```python
from build123d import *

# Parameters (mm, degrees)
F0_W             = 25
F0_H             = 25
F0_R             = 4
F1_DEPTH         = 3
F2_W             = 10
F2_H             = 0.5
F3_DEPTH         = 6.001
F3_COPIES2_COUNT = 2
F4_R             = 0.24999


# Not quite as in the source:
# - a fillet or chamfer is up to 0.001 mm smaller than in the source, because OpenCascade refuses the exact size
# - a pattern or mirror of a feature is missing from the dataset's text; its kind, count and spacing are read off the source's solid


with BuildPart() as f1:
    # F0 (on Front) → F1 (new body, symmetric)
    with BuildSketch(Plane.XZ):
        Rectangle(F0_W, F0_H)
        Circle(F0_R, mode=Mode.SUBTRACT)
    extrude(amount=F1_DEPTH, both=True)

    # F2 (on face) → F3 (cut, through all)
    with BuildSketch(Plane.XZ.offset(3)):
        with BuildLine():
            ThreePointArc((-4.2426406871, 4.2426406871), (-2.2961005942, 5.5432771951), (0, 6))
            Line((0, 6), (0, 6.5))
            ThreePointArc((0, 6.5), (-1.96297305, 6.1965100504), (-3.7426406871, 5.3143805554))
            Line((-3.7426406871, 5.3143805554), (-3.7426406871, 9.75))
            Line((-3.7426406871, 9.75), (-4.2426406871, 9.75))
            Line((-4.2426406871, 9.75), (-4.2426406871, 4.2426406871))
        make_face()
        with BuildLine():
            Line((-6.5, 0), (-6, 0))
            ThreePointArc((-6, 0), (-5.6105188763, 2.1265177965), (-4.4926406871, 3.9769560793))
            Line((-4.4926406871, 3.9769560793), (-4.4926406871, 9.75))
            Line((-4.4926406871, 9.75), (-10, 9.75))
            Line((-10, 9.75), (-10, 9.25))
            Line((-10, 9.25), (-4.9926406871, 9.25))
            Line((-4.9926406871, 9.25), (-4.9926406871, 4.1621555677))
            ThreePointArc((-4.9926406871, 4.1621555677), (-6.1115531768, 2.2133498971), (-6.5, 0))
        make_face()
        with Locations((-5, 10.25)):
            Rectangle(F2_W, F2_H)
    f3 = extrude(amount=-F3_DEPTH, mode=Mode.SUBTRACT)

    # F3_copies: F3 across plane
    add(f3.mirror(Plane(origin=(0, 0, 0), x_dir=(-1, 0, 0), z_dir=(0, 0, -1))), mode=Mode.SUBTRACT)

    # F3_copies1: F3 across plane
    add(f3.mirror(Plane(origin=(0, 0, 0), x_dir=(0, 0, 1), z_dir=(1, 0, 0))), mode=Mode.SUBTRACT)

    # F3_copies2: F3 ×2 about axis
    f3_copies2_axis = Axis((0, 0, 0), (0, 1, 0))
    for i in range(1, F3_COPIES2_COUNT):
        add(f3.rotate(f3_copies2_axis, i * 360 / F3_COPIES2_COUNT), mode=Mode.SUBTRACT)

    # F4 (radius 0.25 in the source; OpenCascade refuses exactly that, so slightly less here)
    f4_edges = [f1.edges().sort_by_distance(p)[0] for p in [
        (-10, 0, 10),
        (-4.492641, 0, 9.75),
        (-4.492641, 0, 3.976956),
        (-4.242641, 0, 4.242641),
        (-10, 0, 10.5),
        (-4.242641, 0, 9.75),
        (-10, 0, 9.25),
        (-10, 0, 9.75),
        (-3.742641, 0, 9.75),
        (-3.742641, 0, 5.314381),
        (10, 0, 10),
        (10, 0, 10.5),
        (10, 0, 9.25),
        (10, 0, 9.75),
        (4.492641, 0, 9.75),
        (4.492641, 0, 3.976956),
        (4.492641, 0, -3.976956),
        (4.492641, 0, -9.75),
        (10, 0, -9.75),
        (10, 0, -9.25),
        (4.242641, 0, 4.242641),
        (4.242641, 0, 9.75),
        (3.742641, 0, 9.75),
        (3.742641, 0, 5.314381),
        (-10, 0, -9.25),
        (-10, 0, -9.75),
        (-4.492641, 0, -9.75),
        (-4.492641, 0, -3.976956),
        (-3.742641, 0, -9.75),
        (-3.742641, 0, -5.314381),
        (3.742641, 0, -5.314381),
        (3.742641, 0, -9.75),
        (4.242641, 0, -9.75),
        (4.242641, 0, -4.242641),
        (-4.242641, 0, -4.242641),
        (-4.242641, 0, -9.75),
        (10, 0, -10),
        (10, 0, -10.5),
        (-10, 0, -10),
        (-10, 0, -10.5),
    ]]
    fillet(f4_edges, radius=F4_R)


solid = f1.part
```
Work out the finished part from the listing and answer in its coordinate system (mm). A direction names the side the tool comes from. Give positions to 0.01 mm unless a question says otherwise; leave off trailing zeros. Write each loop counter-clockwise with the first axis right and the second up, starting at its lowest first coordinate (ties: lowest second). Pieces come first, ordered by that corner, then holes. Notation, with made-up numbers: (-11, 84.25) -> (17, 84.25) arc R12 ccw to (17, 106.25) -> close; hole circle Ø8 at (25.25, 8.25). An arc over 180 degrees is marked (long way). Write each question's results on one line, items separated by ' | '.
1. Find section A-A on z = 7.5. Determine the outline of the cut face in (x, y).
Data:
outline: (-12.5, -3) -> (-4.99, -3) -> (-4.99, 3) -> (-12.5, 3) -> close; (-4.49, -3) -> (-4.24, -3) -> (-4.24, 3) -> (-4.49, 3) -> close; (-3.74, -3) -> (3.74, -3) -> (3.74, 3) -> (-3.74, 3) -> close; (4.24, -3) -> (4.49, -3) -> (4.49, 3) -> (4.24, 3) -> close; (4.99, -3) -> (12.5, -3) -> (12.5, 3) -> (4.99, 3) -> close
2. Find section D-D on y = 0.35. Give the number of separate pieces and of enclosed holes in the cut face, and give its area (3 significant figures).
Data:
separate pieces: 1 | enclosed holes: 7 | area: 506 mm^2
3. Find section B-B on x = -1.75. Determine the outline of the cut face in (y, z).
Data:
outline: (-3, -12.5) -> (3, -12.5) -> (3, -10.5) -> (-3, -10.5) -> close; (-3, -10) -> (3, -10) -> (3, -6.26) -> (-3, -6.26) -> close; (-3, -5.74) -> (3, -5.74) -> (3, -3.6) -> (-3, -3.6) -> close; (-3, 3.6) -> (3, 3.6) -> (3, 5.74) -> (-3, 5.74) -> close; (-3, 6.26) -> (3, 6.26) -> (3, 10) -> (-3, 10) -> close; (-3, 10.5) -> (3, 10.5) -> (3, 12.5) -> (-3, 12.5) -> close
4. A tool of negligible diameter and unlimited length cuts with its end or side. For faces 1 (the flat face through (-3, 3, 3)), 2 (the flat face through (7, 0, 9.25)), from which of +Z, -Z, +X, -X, +Y, -Y can it reach the whole face along a straight path? Write none if from no direction.
Data:
face 1: +Z, -Z, +X, -X, +Y | face 2: +Y, -Y
5. Find section C-C on z = -1.5. Determine the outline of the cut face in (x, y).
Data:
outline: (-12.5, -3) -> (-6.32, -3) -> (-6.32, 3) -> (-12.5, 3) -> close; (-5.81, -3) -> (-3.71, -3) -> (-3.71, 3) -> (-5.81, 3) -> close; (3.71, -3) -> (5.81, -3) -> (5.81, 3) -> (3.71, 3) -> close; (6.32, -3) -> (12.5, -3) -> (12.5, 3) -> (6.32, 3) -> close
6. Determine the mould class of faces 3 (the flat face through (0, 0, 10)), 4 (the flat face through (12.5, 0, 0)) for opening direction Z: +Z half, -Z half, draft (parallel to the pull), parting line (faces both ways), or undercut.
Data:
face 3: undercut | face 4: draft
7. Straight lines are drawn through the part: L1, parallel to X at y = 2.55, z = 7.5; L2, parallel to Z at x = 9.5, y = -1.2; L3, parallel to X at y = -0.65, z = -0.25. For each, find the intervals that lie inside material, in ascending order.
Data:
L1: -12.5 to -4.99, -4.49 to -4.24, -3.74 to 3.74, 4.24 to 4.49, 4.99 to 12.5 | L2: -12.5 to -10.5, -10 to -9.75, -9.25 to 9.25, 9.75 to 10, 10.5 to 12.5 | L3: -12.5 to -6.5, -5.99 to -3.99, 3.99 to 5.99, 6.5 to 12.5
